Read the model definition and answer for the solid it produces. Units are mm, in the model's axes. Coordinates: 2 decimals unless noted, no trailing zeros. Order: outer loops, then holes, each group sorted by start corner. A loop starts at its lowest first (then second) coordinate and runs counter-clockwise, first axis right, second up.
```python
from build123d import *

# Parameters (mm, degrees)
ESQUISSE1_R        = 3
BOSS_EXTRU_1_DEPTH = 5


with BuildPart() as part:
    # Esquisse1 → Boss.-Extru.1 (new body)
    with BuildSketch(Plane.XY.offset(5)):
        with BuildLine():
            Line((-26, 1), (-26, -1))
            ThreePointArc((-26, -1), (-24.535533906, -4.535533906), (-21, -6))
            Line((-21, -6), (21, -6))
            ThreePointArc((21, -6), (24.535533906, -4.535533906), (26, -1))
            Line((26, -1), (26, 1))
            ThreePointArc((26, 1), (24.535533906, 4.535533906), (21, 6))
            Line((21, 6), (-21, 6))
            ThreePointArc((-21, 6), (-24.535533906, 4.535533906), (-26, 1))
        make_face()
        with Locations(Location((21, 0, 0), (0, 0, 180))):  # turned: the seam where the file's is
            Circle(ESQUISSE1_R, mode=Mode.SUBTRACT)
        with Locations(Location((-21, 0, 0), (0, 0, 180))):  # turned: the seam where the file's is
            Circle(ESQUISSE1_R, mode=Mode.SUBTRACT)
    extrude(amount=-BOSS_EXTRU_1_DEPTH)


solid = part.part
```
1) Flat-ended cylindrical pins translate along their axes: pin 1 Ø3.5 at (x, y) = (21, 0) entering from -Z; pin 2 Ø1 at (y, z) = (2, 2) entering from +X. Find the tip coordinate at first contact, or state that the pin passes through.
A:
pin 1: passes through
pin 2: stops at x = 25.97
2) Determine the mould class of faces 1 (the flat face through (0, 0, 5)), 2 (the cylindrical face through (-18, 0, 3)), 3 (the cylindrical face through (25, 4, 3)) for opening direction Y: pulls with the +Y half, pulls with the -Y half, needs draft (parallel to the pull), parting line crosses it, or undercut.
A:
face 1: needs draft
face 2: undercut
face 3: pulls with the +Y half
3) A cutting plane is placed at C-C, the plane y = 4. Determine the outline of the cut face in (x, z), and give its area (3 significant figures).
A:
outline: (-25, 0) - (25, 0) - (25, 5) - (-25, 5) - close
area: 250 mm2
4) Straight lines are drawn through the part: line 1 (X direction, y = -1.75, z = 1.9); line 2 (Y direction, x = -21, z = 2.7); line 3 (X direction, y = -1, z = 3.4). For each, find the intervals that lie inside material, in ascending order.
A:
line 1: x = -25.94 to -23.44, -18.56 to 18.56, 23.44 to 25.94
line 2: y = -6 to -3, 3 to 6
line 3: x = -26 to -23.83, -18.17 to 18.17, 23.83 to 26
5) A cutting plane is placed at D-D, the plane y = -2.5. Determine the outline of the cut face in (x, z), and give its area (3 significant figures).
A:
outline: (-25.77, 0) - (-22.66, 0) - (-22.66, 5) - (-25.77, 5) - close; (-19.34, 0) - (19.34, 0) - (19.34, 5) - (-19.34, 5) - close; (22.66, 0) - (25.77, 0) - (25.77, 5) - (22.66, 5) - close
area: 225 mm2
6) A cutting plane is placed at B-B, the plane z = 1.3. Determine the outline of the cut face in (x, y), and give its area (3 significant figures).
A:
outline: (-26, -1) arc R5 ccw to (-21, -6) - (21, -6) arc R5 ccw to (26, -1) - (26, 1) arc R5 ccw to (21, 6) - (-21, 6) arc R5 ccw to (-26, 1) - close; hole circle Ø6 at (-21, 0); hole circle Ø6 at (21, 0)
area: 546 mm2
7) A cutting plane is placed at A-A, the plane y = 0. Determine the outline of the cut face in (x, z), and give its area (3 significant figures).
A:
outline: (-26, 0) - (-24, 0) - (-24, 5) - (-26, 5) - close; (-18, 0) - (18, 0) - (18, 5) - (-18, 5) - close; (24, 0) - (26, 0) - (26, 5) - (24, 5) - close
area: 200 mm2
